```python
from build123d import *

# Parameters (mm, degrees)
YAW_ARM_BASE_DEPTH           = 4
YAW_ARM_MOUNTING_HOLE_REACH  = 35.29
SKETCH2_R                    = 3.75
YAW_ARM_SLOT_DEPTH           = 1.9
SKETCH5_W                    = 12
SKETCH5_H                    = 4
MOUNTING_BRACKET_DEPTH       = 14
BRACKET_MOUNTING_HOLES_REACH = 39.713
SKETCH8_R                    = 1.125
F_1MM_FILLETS_R              = 1


with BuildPart() as part:
    # Sketch1 → Yaw Arm Base (new body)
    with BuildSketch(Plane(origin=(0, 0, 0), x_dir=(1, 0, 0), z_dir=(0, 1, 0))):
        with BuildLine():
            Line((-6, 0), (-6, -32.5))
            Line((-6, -32.5), (6, -32.5))
            Line((6, -32.5), (6, 0))
            ThreePointArc((6, 0), (0, 6), (-6, 0))
        make_face()
    extrude(amount=YAW_ARM_BASE_DEPTH)

    # Sketch2 → Yaw Arm Mounting Hole (cut, up to next)
    with BuildSketch(Plane(origin=(0, 4, 0), x_dir=(1, 0, 0), z_dir=(0, 1, 0)), mode=Mode.PRIVATE) as yaw_arm_mounting_hole_sk1:
        with Locations(Location((0, 0, 0), (0, 0, 270))):
            Circle(SKETCH2_R)
    yaw_arm_mounting_hole_tool1 = extrude(yaw_arm_mounting_hole_sk1.sketch, amount=-YAW_ARM_MOUNTING_HOLE_REACH, mode=Mode.PRIVATE) & part.part
    add(yaw_arm_mounting_hole_tool1.solids().sort_by_distance((0, 4, 0))[0], mode=Mode.SUBTRACT)

    # Sketch4 → Yaw Arm Slot (cut)
    with BuildSketch(Plane(origin=(0, 4, 0), x_dir=(1, 0, 0), z_dir=(0, 1, 0))):
        with BuildLine():
            Line((-3.46, -1.445994467), (-1.989882432, -16.005994467))
            ThreePointArc((-1.989882432, -16.005994467), (0, -17.805076808), (1.989882432, -16.005994467))
            Line((1.989882432, -16.005994467), (3.46, -1.445994467))
            ThreePointArc((3.46, -1.445994467), (0, -3.75), (-3.46, -1.445994467))
        make_face()
    extrude(amount=-YAW_ARM_SLOT_DEPTH, mode=Mode.SUBTRACT)

    # Sketch5 → Mounting Bracket (add)
    with BuildSketch(Plane.XZ):
        with Locations((0, 30.5)):
            Rectangle(SKETCH5_W, SKETCH5_H)
    extrude(amount=MOUNTING_BRACKET_DEPTH)

    # Sketch8 → Bracket Mounting Holes (cut, up to next)
    with BuildSketch(Plane(origin=(0, 0, 28.5), x_dir=(-1, 0, 0), z_dir=(0, 0, -1)), mode=Mode.PRIVATE) as bracket_mounting_holes_sk1:
        with Locations((-2.5, -10)):
            Circle(SKETCH8_R)
    bracket_mounting_holes_tool1 = extrude(bracket_mounting_holes_sk1.sketch, amount=-BRACKET_MOUNTING_HOLES_REACH, mode=Mode.PRIVATE) & part.part
    # Sketch8 → Bracket Mounting Holes (cut, up to next)
    with BuildSketch(Plane(origin=(0, 0, 28.5), x_dir=(-1, 0, 0), z_dir=(0, 0, -1)), mode=Mode.PRIVATE) as bracket_mounting_holes_sk2:
        with Locations((2.5, -7)):
            Circle(SKETCH8_R)
    bracket_mounting_holes_tool2 = extrude(bracket_mounting_holes_sk2.sketch, amount=-BRACKET_MOUNTING_HOLES_REACH, mode=Mode.PRIVATE) & part.part
    add(bracket_mounting_holes_tool1.solids().sort_by_distance((2.5, -10, 28.5))[0], mode=Mode.SUBTRACT)
    add(bracket_mounting_holes_tool2.solids().sort_by_distance((-2.5, -7, 28.5))[0], mode=Mode.SUBTRACT)

    # 1mm Fillets
    f_1mm_fillets_edges = [part.edges().sort_by_distance(p)[0] for p in [
        (0, 4, 32.5),
        (6, 4, 16.25),
        (6, 0, 14.25),
        (0, 0, 28.5),
        (-6, -7, 28.5),
        (6, -7, 28.5),
        (-6, -14, 30.5),
        (0, -14, 28.5),
        (6, -14, 30.5),
        (0, -14, 32.5),
        (0, 4, -6),
        (-6, 0, 14.25),
        (0, 0, -6),
        (6, -5, 32.5),
        (-6, -5, 32.5),
        (-6, 4, 16.25),
    ]]
    fillet(f_1mm_fillets_edges, radius=F_1MM_FILLETS_R)


solid = part.part
```
Design review of the part built by this model. Coordinates are the model's own, in mm. A direction names the side the tool comes from. Coordinates: 2 decimals unless noted, no trailing zeros. Write each loop counter-clockwise with the first axis right and the second up, starting at its lowest first coordinate (ties: lowest second). Pieces come first, ordered by that corner, then holes.
1) Mouldability with a two-part tool opening along Z and no side actions: class faces 5 (the cylindrical face through (-5.699, 3.715, 15.97)), 6 (the cylindrical face through (0.165, 1.584, -3.746)), 7 (the cylindrical face through (-0.041, 3.063, 17.805)), 8 (the flat face through (0, -5, 32.5)) as +Z half, -Z half, draft (parallel to the pull), parting line (faces both ways), or undercut.
2) Add section C-C (x = 0). Write out the cut boundary in (y, z).
3) Machinability: for faces 1 (the cylindrical face through (5.699, 3.715, 15.529)), 2 (the cylindrical face through (5.699, 0.285, 13.558)), 3 (the flat face through (-2.735, 3.063, 8.624)), 4 (the flat face through (0, -7, 28.5)), which of the approach directions +Z, -Z, +X, -X, +Y, -Y give a long, thin tool a straight path to every point of the face, cutting with its end or side? Answer none if there is none.
4) Add section B-B (z = 30). Write out the cut boundary in (x, y) (3 decimals), plus the area to 3 significant figures.
5) Insertion check: pin 1 (3 mm diameter, centred on x = -2.5, y = -7, fed in from +Z); pin 2 (3.5 mm diameter, centred on x = 0, z = 10, fed in from +Y); pin 3 (5 mm diameter, centred on x = 4, y = -3, fed in from -Z); pin 4 (3 mm diameter, centred on x = -1.5, z = 7.5, fed in from -Y). Each pin has a flat end and moves straight along its axis. Give the tip position at first contact, or say it passes through.
6) To check wall thickness, follow L1, parallel to Y at x = -2.5, z = 30.55 (3 decimals); L2, parallel to Y at x = 2.5, z = 30.45 (3 decimals); L3, parallel to X at y = 1.7, z = 0. State the ranges of each line that lie inside material, in increasing order.
7) Add section D-D (z = 24.5). Write out the cut boundary in (x, y), plus the area to 3 significant figures.
8) Add section A-A (y = -7). Write out the cut boundary in (x, z) (3 decimals).
Check result:
1. face 5: draft
1. face 6: undercut
1. face 7: undercut
1. face 8: +Z half
2. outline: (-14, 29.5) arc R1 ccw to (-13, 28.5) - (-1, 28.5) arc R1 cw to (0, 27.5) - (0, 3.75) - (2.1, 3.75) - (2.1, 17.81) - (4, 17.81) - (4, 31.5) arc R1 ccw to (3, 32.5) - (-13, 32.5) arc R1 ccw to (-14, 31.5) - close; (0, -5) arc R1 ccw to (1, -6) - (3, -6) arc R1 ccw to (4, -5) - (4, -3.75) - (0, -3.75) - close
3. face 1: +Z, -Z, +X, +Y
3. face 2: -Z, +X, -Y
3. face 3: +Y
3. face 4: -Z, +X, -X, -Y
4. outline: (-6, -13) arc R1 ccw to (-5, -14) - (5, -14) arc R1 ccw to (6, -13) - (6, 3) arc R1 ccw to (5, 4) - (-5, 4) arc R1 ccw to (-6, 3) - close; hole circle Ø2.25 at (-2.5, -7); hole circle Ø2.25 at (2.5, -10)
4. area: 207 mm2
5. pin 1: stops at z = 32.5
5. pin 2: stops at y = 2.1
5. pin 3: stops at z = 28.37
5. pin 4: stops at y = 0
6. L1: y = -14 to -8.125, -5.875 to 4
6. L2: y = -14 to -11.125, -8.875 to 4
6. L3: x = -6 to -3.75, 3.75 to 6
7. outline: (-6, 1) arc R1 ccw to (-5, 0) - (5, 0) arc R1 ccw to (6, 1) - (6, 3) arc R1 ccw to (5, 4) - (-5, 4) arc R1 ccw to (-6, 3) - close
7. area: 47.1 mm2
8. outline: (-6, 29.5) arc R1 ccw to (-5, 28.5) - (-3.625, 28.5) - (-3.625, 32.5) - (-5, 32.5) arc R1 ccw to (-6, 31.5) - close; (-1.375, 28.5) - (5, 28.5) arc R1 ccw to (6, 29.5) - (6, 31.5) arc R1 ccw to (5, 32.5) - (-1.375, 32.5) - close
